Autodesk Inventor part; units mm, degrees
ref_plane "YZ Plane" through (0, 0, 0) normal (1, 0, 0) x (0, 1, 0)
ref_plane "XZ Plane" through (0, 0, 0) normal (0, 1, 0) x (-1, 0, 0)
ref_plane "XY Plane" through (0, 0, 0) normal (0, 0, 1) x (1, 0, 0)
sketch "Sketch5" plane through (0, 0, 0) normal (0, 1, 0) x (-1, 0, 0)
  line L0 (50, 113) -> (-50, 113)
  line L1 (-50, 113) -> (-50, -113)
  line L2 (-50, -113) -> (50, -113)
  line L3 (50, -113) -> (50, 113)
  point P0 (0, 0)
  point P1 (50, 0)
  point P2 (0, 113)
  dimension "d8" = 100
  dimension "d9" = 226
extrude "Extrusion5" add sketch "Sketch5" along normal blind 215
sketch "Sketch9" plane through (-50, 0, -113) normal (-1, 0, 0) x (0, 0, 1)
  line L0 (0, 215) -> (226, 215)
  line L1 (170, 180.25) -> (170, 145.25) construction
  line L2 (163.75, 180.25) -> (163.75, 145.25)
  line L3 (176.25, 145.25) -> (176.25, 180.25)
  arc A0 (176.25, 180.25) -> (163.75, 180.25) centre (170, 180.25) ccw
  arc A1 (163.75, 145.25) -> (176.25, 145.25) centre (170, 145.25) ccw
  line L4 (113, 215) -> (113, 186.8149) construction
  line L5 (56, 180.25) -> (56, 145.25) construction
  line L6 (62.25, 180.25) -> (62.25, 145.25)
  line L7 (49.75, 145.25) -> (49.75, 180.25)
  arc A2 (62.25, 180.25) -> (49.75, 180.25) centre (56, 180.25) ccw
  arc A3 (49.75, 145.25) -> (62.25, 145.25) centre (56, 145.25) ccw
  line L8 (180, 145.25) -> (180, 180.25)
  arc A4 (180, 180.25) -> (160, 180.25) centre (170, 180.25) ccw
  line L9 (160, 180.25) -> (160, 145.25)
  arc A5 (160, 145.25) -> (180, 145.25) centre (170, 145.25) ccw
  line L10 (46, 145.25) -> (46, 180.25)
  arc A6 (66, 180.25) -> (46, 180.25) centre (56, 180.25) ccw
  line L11 (66, 180.25) -> (66, 145.25)
  arc A7 (46, 145.25) -> (66, 145.25) centre (56, 145.25) ccw
  circle A8 centre (170, 145.25) radius 9
  point P0 (113, 0)
  point P1 (170, 162.75)
  point P2 (56, 162.75)
  dimension "d41" = 34.75
  dimension "d42" = 35
  dimension "d44" = 114
  dimension "d45" = 57
  dimension "d46" = 12.5
  dimension "d47" = 20
  dimension "d93" = 18
extrude "Extrusion7" cut sketch "Sketch9" against normal through all contours A0 L3 A8 L2 | A8 L3 A1 L2 | L6 A3 L7 A2 picked at (169.6717, 148.232)
extrude "Extrusion8" cut sketch "Sketch9" against normal blind 60 contours L2 A1 L3 A8 | A5 L9 A4 L8 | L10 A6 L11 A7 picked at (163.2862, 148.9936)
chamfer "Chamfer4" distance 20 angle 45 1 edges at (-50, 215, 0)
sketch "Sketch10" plane through (0, 215, 0) normal (0, 1, 0) x (1, 0, 0)
  circle A0 centre (0, -82.5) radius 6
  circle A1 centre (0, 82.5) radius 6
  circle A2 centre (0, -82.5) radius 10
  circle A3 centre (0, 82.5) radius 10
  line L0 (50, -113) -> (50, 113)
  line L1 (-50, -113) -> (50, -113)
  point P0 (0, 0)
  point P1 (0, -113)
  dimension "d55" = 165
  dimension "d56" = 82.5
  dimension "d57" = 12
  dimension "d58" = 20
  dimension "d92" = 50
hole "Hole2" at (0, 215, 82.5) at (0, 215, -82.5) direction (0, -1, 0) diameter 20 depth 140
sketch "Sketch11" plane through (0, 75, -82.5) normal (0, 1, 0) x (1, 0, 0)
  circle A0 centre (0, 0) radius 10
  circle A1 centre (0, 0) radius 6
  circle A2 centre (0, -165) radius 6
  circle A3 centre (0, -165) radius 10
  circle A4 centre (0, 0) radius 10
  point P0 (0, -82.5)
  dimension "d66" = 12
hole "Hole3" at (0, 75, -82.5) at (0, 75, 82.5) direction (0, -1, 0) diameter 10.106 end through all
sketch "Sketch12" plane through (0, 215, 0) normal (0, 1, 0) x (1, 0, 0)
  circle A0 centre (0, -82.5) radius 10
  line L0 (50, -113) -> (50, 113)
  circle A1 centre (0, 0) radius 6
  point P0 (50, 0)
  dimension "d74" = 12
hole "Hole4" at (0, 215, 0) direction (0, -1, 0) diameter 10.106 depth 30 tip angle 118
sketch "Sketch13" plane through (-50, 0, -113) normal (-1, 0, 0) x (0, 0, 1)
  line L0 (0, 0) -> (226, 0)
  circle A0 centre (113, 107.5) radius 6
  line L1 (0, 0) -> (0, 215)
  line L2 (226, 215) -> (0, 215)
  point P0 (113, 0)
  point P1 (0, 107.5)
  point P2 (113, 0)
  dimension "d82" = 12
  dimension "d83" = 107.5
hole "Hole5" at (-50, 107.5, 0) direction (1, 0, 0) diameter 10.106 depth 30 tip angle 118
chamfer "Chamfer5" distance 1 angle 45 13 edges at (-50, 97.5, 113) (-40, 205, 113) (10, 215, 113) (10, 215, -113) (-40, 205, -113) (-50, 97.5, -113) (0, 0, -113) (0, 0, 113) (50, 107.5, 113) (50, 107.5, -113) (50, 215, 0) (50, 0, 0) (-50, 0, 0)
sketch "Sketch14" plane through (-50, 1, -112) normal (-1, 0, 0) x (0, 0, 1)
  line L0 (225, -1) -> (216, -1)
  line L1 (216, -1) -> (216, 9)
  line L2 (216, 9) -> (225, 9)
  line L3 (225, 9) -> (225, -1)
  line L4 (225, 0) -> (225, 193.5858)
  line L5 (0, -1) -> (224, -1)
  line L6 (112, -1) -> (112, -17.0176) construction
  line L7 (-1, -1) -> (8, -1)
  line L8 (8, -1) -> (8, 9)
  line L9 (8, 9) -> (-1, 9)
  line L10 (-1, 9) -> (-1, -1)
  point P0 (-1, 0)
  dimension "d97" = 10
  dimension "d98" = 9
extrude "Extrusion9" cut sketch "Sketch14" against normal through all
chamfer "Chamfer6" distance 1 angle 45 4 edges at (0, 10, 113) (0, 0, 104) (0, 0, -104) (0, 10, -113)
properties part number "BC-10009" material "Aço Carbono AISI 1006"
Can you work these out from the model? Positions are in its coordinate system, mm. A direction names the side the tool comes from. Give positions to 0.01 mm unless a question says otherwise; leave off trailing zeros. Order: outer loops, then holes, each group sorted by start corner. A loop starts at its lowest first (then second) coordinate and runs counter-clockwise, first axis right, second up. Notation, with made-up numbers: M 34,71 L 60,71 A20 ccw 60,79 Z; hole C 53.5,87.5 d2. An arc over 180 degrees is marked long. One line per item, written item: value.
Item 1: For faces 1 (the face through (30, 163, -63.25)), 2 (the face through (-5, 75, -85)), 3 (the face through (-39.791, 204.511, -112.493)), 4 (the face through (50, 106, 2)), 5 (the face through (-34.79, 102.49, -0.66)), which set-ups out of +Z, -Z, +X, -X, +Y, -Y let a thin tool reach every point of the face, with its end or its side?
Verdict:
face 1: +X, -X
face 2: +Y
face 3: -Z, -X, +Y
face 4: +Z, -Z, +X, +Y, -Y
face 5: -X
Item 2: If we section it at D-D on z = -82.5: Write out the boundary of the cut face in (x, y), and give its area (3 significant figures).
Verdict:
outline: M -50,1 L -49,0 L -5.05,0 L -5.05,75 L -10,75 L -10,215 L -30,215 L -50,195 Z; M 5.05,0 L 49,0 L 50,1 L 50,214 L 49,215 L 10,215 L 10,75 L 5.05,75 Z
area: 17,700 mm2
Item 3: If we mould it in two halves opening along Y, with no side actions, what happens to faces 6 (the face through (-20.42, 135.252, -57.22)), 7 (the face through (-0.44, 144.02, 72.51)), 8 (the face through (-1, 10, -108))? For each: pulls with the +Y half, pulls with the -Y half, needs draft (parallel to the pull), parting line crosses it, or undercut.
Verdict:
face 6: undercut
face 7: needs draft
face 8: pulls with the -Y half
Item 4: If we section it at B-B on x = 31.5: Write out the boundary of the cut face in (y, z).
Verdict:
outline: M 0,-103 L 1,-104 L 10,-104 L 10,-112 L 11,-113 L 214,-113 L 215,-112 L 215,112 L 214,113 L 11,113 L 10,112 L 10,104 L 1,104 L 0,103 Z; hole M 145.25,-63.25 L 180.25,-63.25 A6.25 ccw 180.25,-50.75 L 145.25,-50.75 A6.25 ccw Z; hole M 145.25,50.75 L 180.25,50.75 A6.25 ccw 180.25,63.25 L 145.25,63.25 A6.25 ccw Z
Item 5: Please list where these lines run through material, in increasing order: line 1 (Z direction, x = 0, y = 41); line 2 (X direction, y = 31, z = -82.5); line 3 (Z direction, x = 0, y = 115.5).
Verdict:
line 1: -113 to -87.55, -77.45 to 77.45, 87.55 to 113
line 2: -50 to -5.05, 5.05 to 50
line 3: -113 to -92.5, -72.5 to 72.5, 92.5 to 113
Item 6: For pin 1 (11.5 mm diameter, centred on x = 0, z = -82.5, fed in from -Y); pin 2 (2.5 mm diameter, centred on x = 22, y = 6.5, fed in from +Z); pin 3 (10 mm diameter, centred on y = 172, z = 53, fed in from -X); pin 4 (2.5 mm diameter, centred on x = -13, z = 109, fed in from -Y), each with a flat end and sliding along its axis, tell me the tip position at first contact or that it passes through.
Verdict:
pin 1: y = 0
pin 2: z = 104
pin 3: x = 10
pin 4: y = 10
Item 7: If we section it at A-A on z = -57: Write out the boundary of the cut face in (x, y).
Verdict:
outline: M -50,1 L -49,0 L 49,0 L 50,1 L 50,139 L 10,139 L 10,135.25 L -50,135.25 Z; M -50,190.25 L 10,190.25 L 10,186.5 L 50,186.5 L 50,214 L 49,215 L -30,215 L -50,195 Z
Item 8: If we section it at C-C on x = -38: Write out the boundary of the cut face in (y, z), and give its area (3 significant figures).
Verdict:
outline: M 0,-103 L 1,-104 L 10,-104 L 10,-112 L 11,-113 L 205.59,-113 L 207,-112 L 207,112 L 205.59,113 L 11,113 L 10,112 L 10,104 L 1,104 L 0,103 Z; hole C 107.5,0 d10.11; hole M 145.25,-67 L 180.25,-67 A10 ccw 180.25,-47 L 145.25,-47 A10 ccw Z; hole M 145.25,47 L 180.25,47 A10 ccw 180.25,67 L 145.25,67 A10 ccw Z
area: 44,500 mm2
